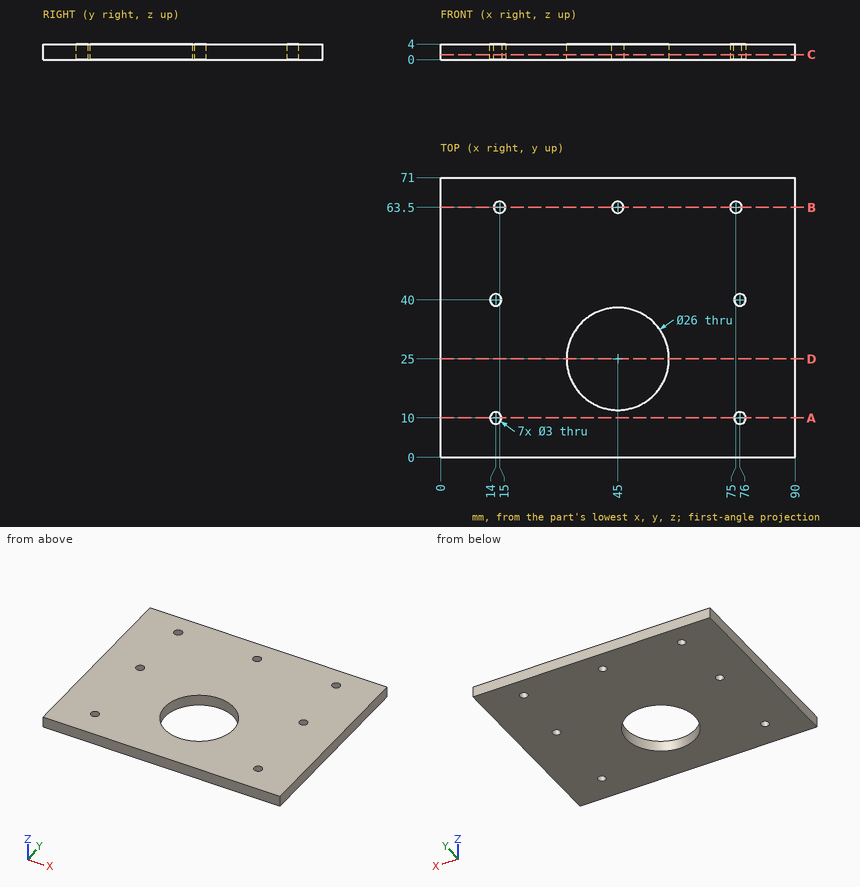
Could you check a few things on this drawing? It's one solid part, dimensions in mm from its lowest x, y, z. Round coordinates to 2 decimals unless told otherwise and drop trailing zeros. Order: outer loops, then holes, each group sorted by start corner. A loop starts at its lowest first (then second) coordinate and runs counter-clockwise, first axis right, second up. Notation, with made-up numbers: M -11,-20.5 L -4,-20.5 A32 cw -4,12.5 Z; hole C 68.25,-15.75 d6. An arc over 180 degrees is marked long. Return JSON: item names as keys, results as strings. Group by question number.
1. If we section it at A-A on y = 10: List the corners of the cut face in (x, z) for me.
2. If we section it at D-D on y = 25: List the corners of the cut face in (x, z) for me.
3. If we section it at B-B on y = 63.5: List the corners of the cut face in (x, z) for me.
4. Please list where these lines run through material, in increasing order: probe 1 along Y at (x, z) = (45, 1.85); probe 2 along X at (y, z) = (63, 3.5); probe 3 along Y at (x, z) = (15, 1.5).
5. If we section it at C-C on z = 1.3: State how many separate pieces and enclosed holes the cut face has, then the cut area to 3 significant figures.
Reply:
{
 "1": {"outline": "M 0,0 L 12.5,0 L 12.5,4 L 0,4 Z; M 15.5,0 L 74.5,0 L 74.5,4 L 15.5,4 Z; M 77.5,0 L 90,0 L 90,4 L 77.5,4 Z"},
 "2": {"outline": "M 0,0 L 32,0 L 32,4 L 0,4 Z; M 58,0 L 90,0 L 90,4 L 58,4 Z"},
 "3": {"outline": "M 0,0 L 13.5,0 L 13.5,4 L 0,4 Z; M 16.5,0 L 43.5,0 L 43.5,4 L 16.5,4 Z; M 46.5,0 L 73.5,0 L 73.5,4 L 46.5,4 Z; M 76.5,0 L 90,0 L 90,4 L 76.5,4 Z"},
 "4": {"probe 1": "0 to 12, 38 to 62, 65 to 71", "probe 2": "0 to 13.59, 16.41 to 43.59, 46.41 to 73.59, 76.41 to 90", "probe 3": "0 to 8.88, 11.12 to 38.88, 41.12 to 62, 65 to 71"},
 "5": {"separate pieces": "1", "enclosed holes": "8", "area": "5,810 mm^2"}
}
